Job drawing, mm, ordinate dimensions from the low corner. One solid piece. Round coordinates to 2 decimals unless told otherwise and drop trailing zeros. Loops run counter-clockwise (first coordinate to the right, second up) from the corner with the lowest first, then second, coordinate; pieces in that order, holes last.
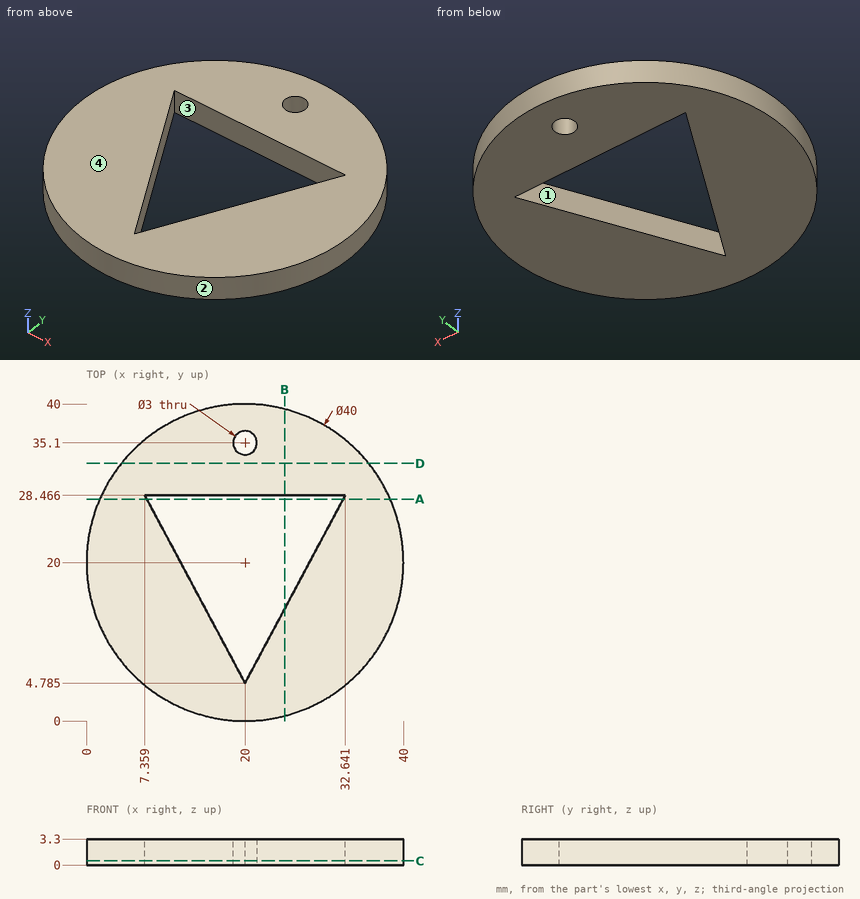
Item 1: Cut at A-A, the plane y = 28. Give the cut face in (x, z).
Answers follow:
outline: (1.67, 0) - (7.61, 0) - (7.61, 3.3) - (1.67, 3.3) - close; (32.39, 0) - (38.33, 0) - (38.33, 3.3) - (32.39, 3.3) - close
Item 2: Two-plate mould, pull along Y, no slides. Class the marked faces 1, 2, 3 and 4: released by +Y, released by -Y, zero draft, split by the parting line, or undercut.
Answers follow:
face 1: undercut
face 2: split by the parting line
face 3: undercut
face 4: zero draft
Item 3: Cut at B-B, the plane x = 25. Give the cut face in (y, z) (1 decimal).
Answers follow:
outline: (0.6, 0) - (14.2, 0) - (14.2, 3.3) - (0.6, 3.3) - close; (28.5, 0) - (39.4, 0) - (39.4, 3.3) - (28.5, 3.3) - close
Item 4: Flat gauge pins, fed straight in: P1, Ø1.5, axis at x = 9, z = 2, coming from the +Y side (1 decimal); P2, Ø1.8, axis at x = 20, y = 35.1, coming from the -Z side. Where does each tip first touch, or does it go through?
Answers follow:
P1: stops at y = 37.2
P2: passes through
Item 5: Probe line 1 (Y direction, x = 22, z = 0.2) (1 decimal); line 2 (X direction, y = 18, z = 3.05) (1 decimal); line 3 (X direction, y = 8, z = 1.45) (1 decimal). List the from-to ranges inside material, lowest first.
Answers follow:
line 1: y = 0.1 to 8.5, 28.5 to 39.9
line 2: x = 0.1 to 12.9, 27.1 to 39.9
line 3: x = 4 to 18.3, 21.7 to 36
Item 6: Cut at D-D, the plane y = 32.5. Give the cut face in (x, z).
Answers follow:
outline: (4.39, 0) - (35.61, 0) - (35.61, 3.3) - (4.39, 3.3) - close
Item 7: Cut at C-C, the plane z = 0.55. Give the cut face in (x, y) (1 decimal).
Answers follow:
outline: circle Ø40 at (20, 20); hole (7.4, 28.5) - (20, 4.8) - (32.6, 28.5) - close; hole circle Ø3 at (20, 35.1)
